Source: three-view drawing plus pictorial views. Frame: mm from the lowest corner of the part. A direction names the side the tool comes from. Coordinates: 2 decimals unless noted, no trailing zeros. Loops run counter-clockwise (first coordinate to the right, second up) from the corner with the lowest first, then second, coordinate; pieces in that order, holes last. Notation, with made-up numbers: M 12,41.5 L 19,41.5 A18 cw 19,60.5 Z; hole C -15,0.5 d7. An arc over 180 degrees is marked long. Use a Markdown table: item, result. Add a question column.
1. Pin query (flat end, axial travel): pin 1 (5 mm diameter, centred on x = 16.5, z = 5.5, fed in from -Y); pin 2 (6.5 mm diameter, centred on x = 7, y = 4.5, fed in from +Z); pin 3 (3 mm diameter, centred on x = 2, z = 5, fed in from +Y). Return the tip coordinate at first contact, or that it passes through.
2. Line query: L1, parallel to Z at x = 4, y = 7; L2, parallel to Z at x = 12.5, y = 15.5; L3, parallel to Y at x = 15.25, z = 7. Output: solid intervals per line, ascending. Write a range as [from, to].
3. Draft query along Z for the marked faces 4, 5 and 6. Return one class per face: +Z half, -Z half, draft (parallel to the pull), parting line (faces both ways), or undercut.
4. Section A-A on y = 15. Output: boundary loops of the cut face in (x, z) (1 decimal).
5. Section D-D on y = 28.5. Output: boundary loops of the cut face in (x, z).
6. Set-up query: the marked faces 1, 2 and 3. Return all of +Z, -Z, +X, -X, +Y, -Y with unobstructed straight access to the full face (end or side cutting, diameter ignored); none if empty.
7. Section B-B on z = 7.75. Output: boundary loops of the cut face in (x, y) (1 decimal).
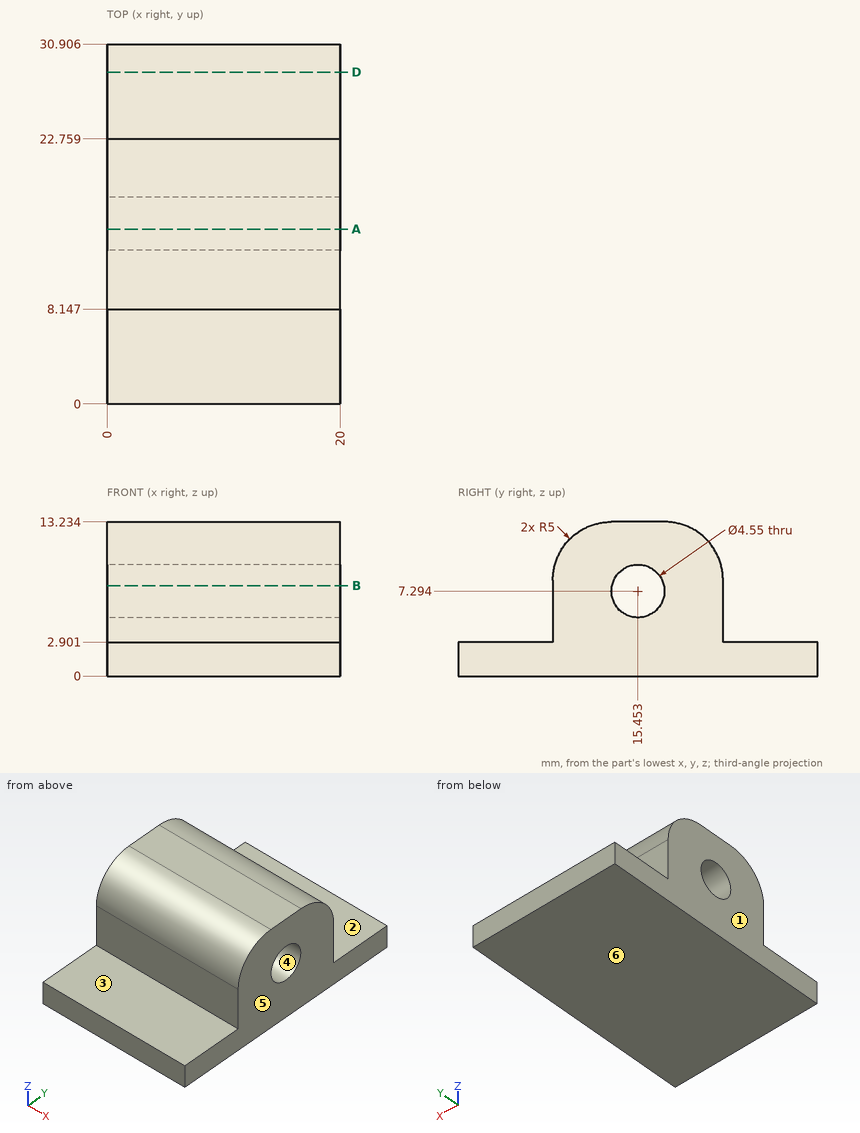
Answers below:
| question | item | result |
|---|---|---|
| 1 | pin 1 | stops at y = 8.15 |
| 1 | pin 2 | stops at z = 2.9 |
| 1 | pin 3 | stops at y = 22.76 |
| 2 | L1 | z = [0, 2.9] |
| 2 | L2 | z = [0, 5.02], [9.57, 13.23] |
| 2 | L3 | y = [8.15, 13.2], [17.71, 22.76] |
| 3 | face 4 | undercut |
| 3 | face 5 | draft |
| 3 | face 6 | -Z half |
| 4 | outline | M 0,0 L 20,0 L 20,5.1 L 0,5.1 Z; M 0,9.5 L 20,9.5 L 20,13.2 L 0,13.2 Z |
| 5 | outline | M 0,0 L 20,0 L 20,2.9 L 0,2.9 Z |
| 6 | face 1 | +Z, -Z, -X, +Y, -Y |
| 6 | face 2 | +Z, +X, -X, +Y |
| 6 | face 3 | +Z, +X, -X, -Y |
| 7 | outline | M 0,8.1 L 20,8.1 L 20,13.2 L 0,13.2 Z; M 0,17.7 L 20,17.7 L 20,22.8 L 0,22.8 Z |
